Verification items for the finished model (mm, model axes). A direction names the side the tool comes from. Give positions to 0.01 mm unless a question says otherwise; leave off trailing zeros. Write each loop counter-clockwise with the first axis right and the second up, starting at its lowest first coordinate (ties: lowest second). Pieces come first, ordered by that corner, then holes. Notation, with made-up numbers: (70.25, 15.25) -> (104.25, 15.25) arc R21 ccw to (104.25, 50.25) -> close; hole circle Ø7 at (65, 59.5). An arc over 180 degrees is marked (long way). Use one line per item in the form item = value. Start each with the question number.
(1) Section check B-B, the plane x = 0. Record the cut outline in (y, z).
(2) Section check A-A, the plane y = 0. Record the cut outline in (x, z), plus the area to 3 significant figures.
(3) Section check D-D, the plane z = 5.5. Record the cut outline in (x, y) (1 decimal), plus the area to 3 significant figures.
(4) Section check C-C, the plane z = 2. Record the cut outline in (x, y) (1 decimal), plus the area to 3 significant figures.
(5) Scan lines: L1, parallel to Z at x = 9.9, y = 0; L2, parallel to Y at x = -7.5, z = 0.5. Record each from-to range of solid material in increasing order.
(6) Depth check by flat-ended pin: pin 1 Ø5 at (x, y) = (-4, 2) entering from -Z; pin 2 Ø1 at (y, z) = (8.5, 4.5) entering from +X; pin 3 Ø1 at (x, z) = (-6, 2) entering from +Y. Enter the tip coordinate at first touch or a pass-through.
(7) Set-up check for faces 4 (the face through (0.19, -11.11, 3.24)), 5 (the face through (0, -6, 4.978)): record each of +Z, -Z, +X, -X, +Y, -Y from which the full face is reachable in a straight line by a thin tool's end or side.
(8) Release check for a two-part mould opening along Z. For faces 1 (the face through (9.46, 0.072, 4.126)), 2 (the face through (-5, 5, 6.566)), 3 (the face through (-10.319, 1, 4)) record: pulls with the +Z half, pulls with the -Z half, needs draft (parallel to the pull), parting line crosses it, or undercut.
Autodesk Inventor part; units mm, degrees
ref_plane "YZ Plane" through (0, 0, 0) normal (1, 0, 0) x (0, 1, 0)
ref_plane "XZ Plane" through (0, 0, 0) normal (0, 1, 0) x (-1, 0, 0)
ref_plane "XY Plane" through (0, 0, 0) normal (0, 0, 1) x (1, 0, 0)
sketch "Sketch1" plane through (0, 0, 0) normal (0, 0, 1) x (1, 0, 0)
  circle A0 centre (0, 0) radius 11.1125
  circle A1 centre (0, 0) radius 6.35
  circle A2 centre (0, 0) radius 8.7313
  dimension "d0" = 22.225
  dimension "d1" = 12.7
  dimension "d34" = 2.3813
  dimension "d35" = 2.3813
extrude "Extrusion3" add sketch "Sketch1" along normal blind 4.9784 contours A0
sketch "Sketch2" plane through (0, 0, 4.9784) normal (0, 0, 1) x (1, 0, 0)
  circle A0 centre (0, 0) radius 11.1125
  circle A1 centre (0, 0) radius 5.5563
  dimension "d36" = 11.1125
extrude "Extrusion4" add sketch "Sketch2" along normal blind 1.5875
sketch "Sketch3" plane through (0, 0, 0) normal (1, 0, 0) x (0, 1, 0)
  line L0 (-8.7313, 4.9784) -> (8.7313, 4.9784)
  line L1 (8.7313, 0) -> (-8.7313, 0)
  line L2 (0, 0) -> (0, 4.9784) construction
  point P0 (0, 2.4892)
hole "Hole2" at (0, 0, 2.4892) direction (-1, 0, 0) diameter 3.2766 end through all
sketch "Sketch4" plane through (0, 0, 0) normal (0, 0, -1) x (-1, 0, 0)
  circle A0 centre (0, 0) radius 11.1125
  line L0 (0, 0) -> (-11.1125, 0) construction
  line L1 (-10.3187, 4.1244) -> (-10.3187, -4.1244)
  circle A1 centre (0, 0) radius 7.9375 construction
  point P0 (-7.9375, 0)
  point P1 (-10.3187, 0)
  dimension "d30" = 15.875
  dimension "d29" = 0.7937
extrude "Extrusion5" cut sketch "Sketch4" against normal through all contours L1 A0 picked at (-10.5166, 0.7)
mirror "Mirror1" about plane through (0, 0, 0) normal (1, 0, 0) of "Hole2", "Extrusion5"
equation "\"d34\" = d35"
properties part number "Pneumatic Connector -Shaft Side Cover"
Completed:
q1.outline = (-11.11, 0) -> (-8.73, 0) -> (-8.73, 4.98) -> (-5.56, 4.98) -> (-5.56, 6.57) -> (-11.11, 6.57) -> close; (5.56, 4.98) -> (8.73, 4.98) -> (8.73, 0) -> (11.11, 0) -> (11.11, 6.57) -> (5.56, 6.57) -> close
q2.outline = (-10.32, 0) -> (-8.73, 0) -> (-8.73, 0.85) -> (-10.32, 0.85) -> close; (-10.32, 4.13) -> (-8.73, 4.13) -> (-8.73, 4.98) -> (-5.56, 4.98) -> (-5.56, 6.57) -> (-10.32, 6.57) -> close; (5.56, 4.98) -> (8.73, 4.98) -> (8.73, 4.13) -> (10.32, 4.13) -> (10.32, 6.57) -> (5.56, 6.57) -> close; (8.73, 0) -> (10.32, 0) -> (10.32, 0.85) -> (8.73, 0.85) -> close
q2.area = 20.5 mm²
q3.outline = (-10.3, -4.1) arc R11.1 ccw to (10.3, -4.1) -> (10.3, 4.1) arc R11.1 ccw to (-10.3, 4.1) -> close; hole circle Ø11.1 at (0, 0)
q3.area = 282 mm²
q4.outline = (-10.3, -4.1) arc R11.1 ccw to (10.3, -4.1) -> (10.3, -1.6) -> (8.6, -1.6) arc R8.7 cw to (-8.6, -1.6) -> (-10.3, -1.6) -> close; (-10.3, 1.6) -> (-8.6, 1.6) arc R8.7 cw to (8.6, 1.6) -> (10.3, 1.6) -> (10.3, 4.1) arc R11.1 ccw to (-10.3, 4.1) -> close
q4.area = 129 mm²
q5.L1 = 0 to 0.85, 4.13 to 6.57
q5.L2 = -8.2 to -4.47, 4.47 to 8.2
q6.pin_1 = 4.98
q6.pin_2 = 7.71
q6.pin_3 = 9.66
q7.face_4 = +Z, -Z, -Y
q7.face_5 = -Z
q8.face_1 = undercut
q8.face_2 = pulls with the +Z half
q8.face_3 = needs draft
